Part model, mm, in its own coordinate system. Round coordinates to 2 decimals unless told otherwise and drop trailing zeros. Write each loop counter-clockwise with the first axis right and the second up, starting at its lowest first coordinate (ties: lowest second). Pieces come first, ordered by that corner, then holes. Notation, with made-up numbers: (54.5, 43.5) -> (98.5, 43.5) arc R16 cw to (98.5, 74.5) -> close; hole circle Ø3 at (-14.5, 38.25). An arc over 180 degrees is marked (long way). Return JSON: item names as keys, results as strings. Group by question number.
(1) Drill centre lines: L1, parallel to Y at x = 0, z = 0.7; L2, parallel to Y at x = 24.5, z = 0.75; L3, parallel to Y at x = -39, z = 1.4. Where is each one in solid material? Low to high. Write a range as from..to.
(2) Saw through at D-D (x = 26). List the corners of the cut face in (y, z), plus the area to 3 significant figures.
(3) Saw through at B-B (z = 0.75). List the corners of the cut face in (x, y).
(4) Saw through at A-A (x = 0). List the corners of the cut face in (y, z), plus the area to 3 significant figures.
(5) Saw through at C-C (y = 0). List the corners of the cut face in (x, z).
(6) Drop flat-ended pins along their axis: pin 1 Ø1 at (x, z) = (44, 0.5) entering from +Y; pin 2 Ø1 at (y, z) = (-43.5, 1) entering from -X; pin 3 Ø1 at (y, z) = (-44.5, 1) entering from +X. Give the stop position or say it passes through.
from build123d import *

# Parameters (mm, degrees)
SKETCH1_R           = 45.85
SKETCH1_R_2         = 10.5
BOSS_EXTRUDE1_DEPTH = 2
CUT_EXTRUDE1_REACH  = 4
SKETCH2_R           = 3
CUT_EXTRUDE2_REACH  = 4


with BuildPart() as part:
    # Sketch1 → Boss-Extrude1 (new body)
    with BuildSketch(Plane.XY):
        Circle(SKETCH1_R)
        Circle(SKETCH1_R_2, mode=Mode.SUBTRACT)
    extrude(amount=BOSS_EXTRUDE1_DEPTH)

    # Sketch2 → Cut-Extrude1 (cut, up to next)
    with BuildSketch(Plane(origin=(0, 0, 0), x_dir=(-1, 0, 0), z_dir=(0, 0, -1)), mode=Mode.PRIVATE) as cut_extrude1_sk1:
        with Locations((-26, 0)):
            Circle(SKETCH2_R)
    cut_extrude1_tool1 = extrude(cut_extrude1_sk1.sketch, amount=-CUT_EXTRUDE1_REACH, mode=Mode.PRIVATE) & part.part
    add(cut_extrude1_tool1.solids().sort_by_distance((26, 0, 0))[0], mode=Mode.SUBTRACT)

    # Sketch3 → Cut-Extrude2 (cut, up to next)
    with BuildSketch(Plane(origin=(0, 0, 0), x_dir=(-1, 0, 0), z_dir=(0, 0, -1)), mode=Mode.PRIVATE) as cut_extrude2_sk1:
        with BuildLine():
            Line((-6, 42.437949998), (-6, 45.455720212))
            ThreePointArc((-6, 45.455720212), (-32.420845917, 32.420845917), (-45.455720212, 6))
            Line((-45.455720212, 6), (-42.437949998, 6))
            ThreePointArc((-42.437949998, 6), (-30.306596642, 30.306596642), (-6, 42.437949998))
        make_face()
    cut_extrude2_tool1 = extrude(cut_extrude2_sk1.sketch, amount=-CUT_EXTRUDE2_REACH, mode=Mode.PRIVATE) & part.part
    add(cut_extrude2_tool1.solids().sort_by_distance((6.557988, 43.946835, 0))[0], mode=Mode.SUBTRACT)
    # Sketch3 → Cut-Extrude2 (cut, up to next)
    with BuildSketch(Plane(origin=(0, 0, 0), x_dir=(-1, 0, 0), z_dir=(0, 0, -1)), mode=Mode.PRIVATE) as cut_extrude2_sk2:
        with BuildLine():
            Line((42.437949998, 6), (45.455720212, 6))
            ThreePointArc((45.455720212, 6), (32.420845917, 32.420845917), (6, 45.455720212))
            Line((6, 45.455720212), (6, 42.437949998))
            ThreePointArc((6, 42.437949998), (30.306596642, 30.306596642), (42.437949998, 6))
        make_face()
    cut_extrude2_tool2 = extrude(cut_extrude2_sk2.sketch, amount=-CUT_EXTRUDE2_REACH, mode=Mode.PRIVATE) & part.part
    add(cut_extrude2_tool2.solids().sort_by_distance((-43.946835, 6.557988, 0))[0], mode=Mode.SUBTRACT)
    # Sketch3 → Cut-Extrude2 (cut, up to next)
    with BuildSketch(Plane(origin=(0, 0, 0), x_dir=(-1, 0, 0), z_dir=(0, 0, -1)), mode=Mode.PRIVATE) as cut_extrude2_sk3:
        with BuildLine():
            Line((6, -42.437949998), (6, -45.455720212))
            ThreePointArc((6, -45.455720212), (32.420845917, -32.420845917), (45.455720212, -6))
            Line((45.455720212, -6), (42.437949998, -6))
            ThreePointArc((42.437949998, -6), (30.306596642, -30.306596642), (6, -42.437949998))
        make_face()
    cut_extrude2_tool3 = extrude(cut_extrude2_sk3.sketch, amount=-CUT_EXTRUDE2_REACH, mode=Mode.PRIVATE) & part.part
    add(cut_extrude2_tool3.solids().sort_by_distance((-32.026289, -32.026289, 0))[0], mode=Mode.SUBTRACT)
    # Sketch3 → Cut-Extrude2 (cut, up to next)
    with BuildSketch(Plane(origin=(0, 0, 0), x_dir=(-1, 0, 0), z_dir=(0, 0, -1)), mode=Mode.PRIVATE) as cut_extrude2_sk4:
        with BuildLine():
            Line((-42.437949998, -6), (-45.455720212, -6))
            ThreePointArc((-45.455720212, -6), (-32.420845917, -32.420845917), (-6, -45.455720212))
            Line((-6, -45.455720212), (-6, -42.437949998))
            ThreePointArc((-6, -42.437949998), (-30.306596642, -30.306596642), (-42.437949998, -6))
        make_face()
    cut_extrude2_tool4 = extrude(cut_extrude2_sk4.sketch, amount=-CUT_EXTRUDE2_REACH, mode=Mode.PRIVATE) & part.part
    add(cut_extrude2_tool4.solids().sort_by_distance((6.557988, -43.946835, 0))[0], mode=Mode.SUBTRACT)


solid = part.part
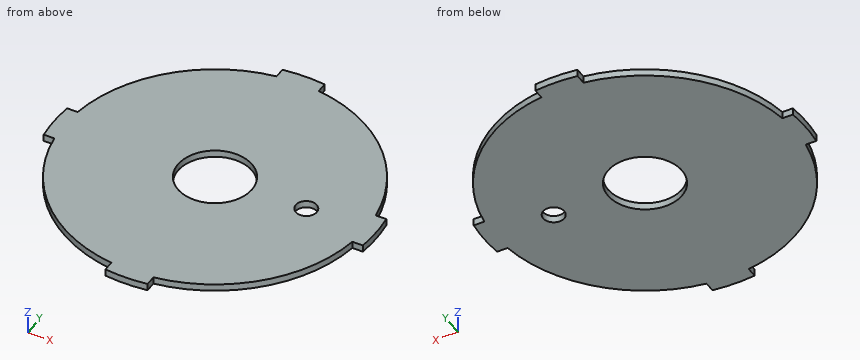
Computed values:
{
 "1": {"L1": "-45.85..-10.5, 10.5..45.85", "L2": "-35.17..-2.6, 2.6..35.17", "L3": "-17.78..17.78"},
 "2": {"outline": "(-34.07, 0) -> (-3, 0) -> (-3, 2) -> (-34.07, 2) -> close; (3, 0) -> (34.07, 0) -> (34.07, 2) -> (3, 2) -> close", "area": "124 mm2"},
 "3": {"outline": "(-45.46, -6) -> (-42.44, -6) arc R42.86 ccw to (-6, -42.44) -> (-6, -45.46) arc R45.85 ccw to (6, -45.46) -> (6, -42.44) arc R42.86 ccw to (42.44, -6) -> (45.46, -6) arc R45.85 ccw to (45.46, 6) -> (42.44, 6) arc R42.86 ccw to (6, 42.44) -> (6, 45.46) arc R45.85 ccw to (-6, 45.46) -> (-6, 42.44) arc R42.86 ccw to (-42.44, 6) -> (-45.46, 6) arc R45.85 ccw to start; hole circle Ø21 at (0, 0); hole circle Ø6 at (26, 0)"},
 "4": {"outline": "(-45.85, 0) -> (-10.5, 0) -> (-10.5, 2) -> (-45.85, 2) -> close; (10.5, 0) -> (45.85, 0) -> (45.85, 2) -> (10.5, 2) -> close", "area": "141 mm2"},
 "5": {"outline": "(-45.85, 0) -> (-10.5, 0) -> (-10.5, 2) -> (-45.85, 2) -> close; (10.5, 0) -> (23, 0) -> (23, 2) -> (10.5, 2) -> close; (29, 0) -> (45.85, 0) -> (45.85, 2) -> (29, 2) -> close"},
 "6": {"pin 1": "y = 6", "pin 2": "x = -6", "pin 3": "x = 6"}
}
